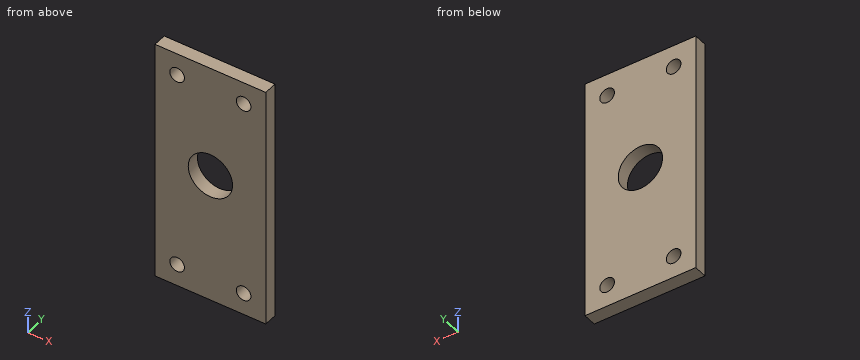
```python
from build123d import *

# Parameters (mm, degrees)
SKETCH_1_W      = 25
SKETCH_1_H      = 55
EXTRUDE_1_DEPTH = 3
HOLE_WIZARD_1_D = 3.3
HOLE_WIZARD_2_D = 10


with BuildPart() as part:
    # 草图1 → 凸台-拉伸1 (new body)
    with BuildSketch(Plane(origin=(0, 0, 0), x_dir=(1, 0, 0), z_dir=(0, 1, 0))):
        Rectangle(SKETCH_1_W, SKETCH_1_H)
    extrude(amount=EXTRUDE_1_DEPTH)

    # 孔1 (through all)
    with Locations(Plane(origin=(0, 3, 0), x_dir=(1, 0, 0), z_dir=(0, 1, 0))):
        with Locations((-7.5, 22.5), (7.5, 22.5), (7.5, -22.5), (-7.5, -22.5)):
            Hole(HOLE_WIZARD_1_D / 2)

    # 孔2 (through all)
    with Locations(Plane(origin=(0, 3, 0), x_dir=(1, 0, 0), z_dir=(0, 1, 0))):
        with Locations((0, -2)):
            Hole(HOLE_WIZARD_2_D / 2)


solid = part.part
```
Check sheet for the modelled part. Datum: model origin and axes. Units: mm. Round coordinates to 2 decimals unless told otherwise and drop trailing zeros. Order: outer loops, then holes, each group sorted by start corner. A loop starts at its lowest first (then second) coordinate and runs counter-clockwise, first axis right, second up. Notation, with made-up numbers: (88.25, 24) -> (119.25, 24) arc R16 ccw to (119.25, 33) -> close; hole circle Ø2 at (87, 7.5). An arc over 180 degrees is marked (long way). One line per item, written item: value. Start each with the question number.
Q1. Cross-section at D-D (z = -22.5). Record the boundary of the cut face in (x, y).
Q2. Cross-section at B-B (z = 2). Record the boundary of the cut face in (x, y), and give its area (3 significant figures).
Q3. Cross-section at A-A (x = 0). Record the boundary of the cut face in (y, z), and give its area (3 significant figures).
Q4. Thickness scan on line 1 (X direction, y = 0.8, z = 22.5); line 2 (Z direction, x = 7.5, y = 1.5); line 3 (Z direction, x = 0, y = 0.7). Record the ranges inside material, lowest first.
Q5. Cross-section at C-C (y = 0.45). Record the boundary of the cut face in (x, z).
Completed:
1. outline: (-12.5, 0) -> (-9.15, 0) -> (-9.15, 3) -> (-12.5, 3) -> close; (-5.85, 0) -> (5.85, 0) -> (5.85, 3) -> (-5.85, 3) -> close; (9.15, 0) -> (12.5, 0) -> (12.5, 3) -> (9.15, 3) -> close
2. outline: (-12.5, 0) -> (-5, 0) -> (-5, 3) -> (-12.5, 3) -> close; (5, 0) -> (12.5, 0) -> (12.5, 3) -> (5, 3) -> close
2. area: 45.0 mm²
3. outline: (0, -27.5) -> (3, -27.5) -> (3, -3) -> (0, -3) -> close; (0, 7) -> (3, 7) -> (3, 27.5) -> (0, 27.5) -> close
3. area: 135 mm²
4. line 1: x = -12.5 to -9.15, -5.85 to 5.85, 9.15 to 12.5
4. line 2: z = -27.5 to -24.15, -20.85 to 20.85, 24.15 to 27.5
4. line 3: z = -27.5 to -3, 7 to 27.5
5. outline: (-12.5, -27.5) -> (12.5, -27.5) -> (12.5, 27.5) -> (-12.5, 27.5) -> close; hole circle Ø3.3 at (-7.5, -22.5); hole circle Ø3.3 at (-7.5, 22.5); hole circle Ø10 at (0, 2); hole circle Ø3.3 at (7.5, -22.5); hole circle Ø3.3 at (7.5, 22.5)
